Geometry: final body of the model. Coordinates: model frame, mm. Face numbers are marked on the shaded views. A direction names the side the tool comes from. Coordinates: 2 decimals unless noted, no trailing zeros. Loops run counter-clockwise (first coordinate to the right, second up) from the corner with the lowest first, then second, coordinate; pieces in that order, holes last. Notation, with made-up numbers: (79, -27) -> (103, -27) arc R17 cw to (103, -13) -> close; hole circle Ø2 at (59, 77.25). An arc over 180 degrees is marked (long way). One line per item, written item: value. Start each with the question number.
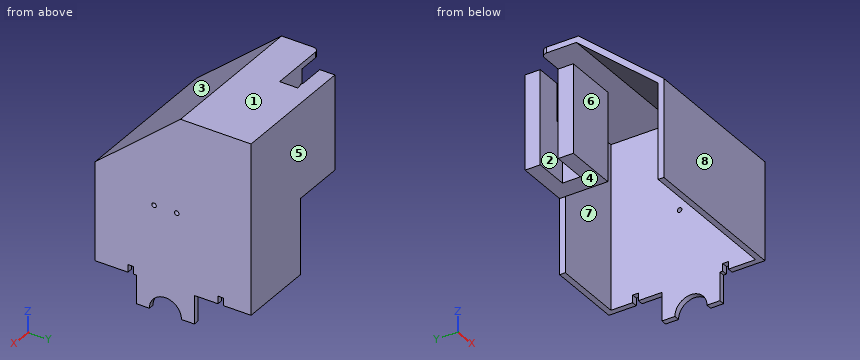
from build123d import *

# Parameters (mm, degrees)
BOSS_EXTRUDE1_DEPTH = 50
SKETCH2_W           = 3
SKETCH2_H           = 22.5
SKETCH2_W_2         = 40
SKETCH2_H_2         = 3
BOSS_EXTRUDE2_DEPTH = 40
SKETCH3_W           = 18
SKETCH3_H           = 9.5
CUT_EXTRUDE1_DEPTH  = 30
SKETCH4_W           = 3
SKETCH4_H           = 90
BOSS_EXTRUDE3_DEPTH = 79.5
SKETCH6_W           = 90
SKETCH6_H           = 3
BOSS_EXTRUDE4_DEPTH = 79
BOSS_EXTRUDE5_DEPTH = 3
FILLET1_R           = 3
SKETCH11_W          = 4
SKETCH11_H          = 3
CUT_EXTRUDE2_DEPTH  = 3
BOSS_EXTRUDE6_DEPTH = 3
SKETCH15_R          = 1.2
SKETCH15_W          = 4
SKETCH15_H          = 3
CUT_EXTRUDE3_DEPTH  = 3
CUT_EXTRUDE4_DEPTH  = 83
BOSS_EXTRUDE7_DEPTH = 82


with BuildPart() as part:
    # Sketch1 → Boss-Extrude1 (new body)
    with BuildSketch(Plane.XY.offset(75.054829109)):
        with BuildLine():
            Line((-97.212578399, 43.970791156), (-83.462578399, 43.970791156))
            ThreePointArc((-83.462578399, 43.970791156), (-82.462578399, 43.470791156), (-81.462578399, 43.970791156))
            Line((-81.462578399, 43.970791156), (-79.212578399, 43.970791156))
            Line((-79.212578399, 43.970791156), (-79.212578399, 34.470791156))
            Line((-79.212578399, 34.470791156), (-97.212578399, 34.470791156))
            Line((-97.212578399, 34.470791156), (-97.212578399, 26.470791156))
            Line((-97.212578399, 26.470791156), (-69.212578399, 26.470791156))
            Line((-69.212578399, 26.470791156), (-69.212578399, 51.970791156))
            Line((-69.212578399, 51.970791156), (-97.212578399, 51.970791156))
            Line((-97.212578399, 51.970791156), (-97.212578399, 43.970791156))
        make_face()
    extrude(amount=BOSS_EXTRUDE1_DEPTH)

    # Sketch2 → Boss-Extrude2 (add)
    with BuildSketch(Plane(origin=(-69.212578399, 0, 0), x_dir=(0, 0, -1), z_dir=(1, 0, 0))):
        with Locations((-123.554829109, 37.720791156)):
            Rectangle(SKETCH2_W, SKETCH2_H)
        Polygon((-75.054829109, 51.970791156), (-125.054829109, 51.970791156), (-125.054829109, 48.970791156), (-122.054829109, 48.970791156), (-75.054829109, 48.970791156), align=None)
        with Locations((-55.054829109, 50.470791156)):
            Rectangle(SKETCH2_W_2, SKETCH2_H_2)
    extrude(amount=BOSS_EXTRUDE2_DEPTH)

    # Sketch3 → Cut-Extrude1 (cut)
    with BuildSketch(Plane(origin=(0, 0, 75.054829109), x_dir=(-1, 0, 0), z_dir=(0, 0, -1))):
        with Locations((88.212578399, 39.220791156)):
            Rectangle(SKETCH3_W, SKETCH3_H)
    extrude(amount=-CUT_EXTRUDE1_DEPTH, mode=Mode.SUBTRACT)

    # Sketch4 → Boss-Extrude3 (add)
    with BuildSketch(Plane.XZ.offset(-48.970791156)):
        with Locations((-30.712578399, 80.054829109)):
            Rectangle(SKETCH4_W, SKETCH4_H)
    extrude(amount=BOSS_EXTRUDE3_DEPTH)

    # Sketch6 → Boss-Extrude4 (add)
    with BuildSketch(Plane.ZY.offset(32.212578399)):
        with Locations((80.054829109, -29.029208844)):
            Rectangle(SKETCH6_W, SKETCH6_H)
    extrude(amount=BOSS_EXTRUDE4_DEPTH)

    # Sketch7 → Boss-Extrude5 (add)
    with BuildSketch(Plane.XY.offset(125.054829109)):
        Polygon((-111.212578399, -27.529208844), (-32.212578399, -27.529208844), (-32.212578399, 26.470791156), (-97.212578399, 26.470791156), (-97.212578399, 34.470791156), (-111.212578399, 34.470791156), align=None)
    extrude(amount=-BOSS_EXTRUDE5_DEPTH)

    # Fillet1
    fillet1_edges = [part.edges().sort_by_distance(p)[0] for p in [
        (-111.212578399, 34.470791156, 123.554829109),
    ]]
    fillet(fillet1_edges, radius=FILLET1_R)

    # Sketch11 → Cut-Extrude2 (cut)
    with BuildSketch(Plane(origin=(-29.212578399, 0, 0), x_dir=(0, 0, -1), z_dir=(1, 0, 0))):
        with Locations((-37.054829109, 35.970791156)):
            Rectangle(SKETCH11_W, SKETCH11_H)
    extrude(amount=-CUT_EXTRUDE2_DEPTH, mode=Mode.SUBTRACT)

    # Sketch13 → Boss-Extrude6 (add)
    with BuildSketch(Plane(origin=(-29.212578399, 0, 0), x_dir=(0, 0, -1), z_dir=(1, 0, 0))):
        with BuildLine():
            Line((-20.054829109, 15.145791156), (-20.054829109, 21.970791156))
            Line((-20.054829109, 21.970791156), (-35.054829109, 21.970791156))
            Line((-35.054829109, 21.970791156), (-35.054829109, -8.679208844))
            Line((-35.054829109, -8.679208844), (-20.054829109, -8.679208844))
            Line((-20.054829109, -8.679208844), (-20.054829109, -1.854208844))
            ThreePointArc((-20.054829109, -1.854208844), (-28.554829109, 6.645791156), (-20.054829109, 15.145791156))
        make_face()
    extrude(amount=-BOSS_EXTRUDE6_DEPTH)

    # Sketch15 → Cut-Extrude3 (cut)
    with BuildSketch(Plane(origin=(-29.212578399, 0, 0), x_dir=(0, 0, -1), z_dir=(1, 0, 0))):
        with Locations((-75.054829109, 0.645791156)):
            Circle(SKETCH15_R)
        with Locations((-75.054829109, 12.645791156)):
            Circle(SKETCH15_R)
        with Locations((-37.054829109, -11.679208844)):
            Rectangle(SKETCH15_W, SKETCH15_H)
    extrude(amount=-CUT_EXTRUDE3_DEPTH, mode=Mode.SUBTRACT)

    # Sketch16 → Cut-Extrude4 (cut, through all)
    with BuildSketch(Plane(origin=(-29.212578399, 0, 0), x_dir=(0, 0, -1), z_dir=(1, 0, 0))):
        Polygon((-125.054829109, 16.970791156), (-85.054829109, -30.529208844), (-125.054829109, -30.529208844), align=None)
    extrude(amount=-CUT_EXTRUDE4_DEPTH, mode=Mode.SUBTRACT)

    # Sketch17 → Boss-Extrude7 (add)
    with BuildSketch(Plane(origin=(-29.212578399, 0, 0), x_dir=(0, 0, -1), z_dir=(1, 0, 0))):
        Polygon((-125.054829109, 19.299492846), (-125.054829109, 14.642089465), (-87.015841059, -30.529208844), (-83.093817159, -30.529208844), align=None)
    extrude(amount=-BOSS_EXTRUDE7_DEPTH)


solid = part.part
1. Section D-D on x = -49. Return the cut outline in (y, z).
2. Section C-C on z = 103. Return the cut outline in (x, y).
3. Set-up query: the marked faces 4, 5, 6, 7 and 8. Return all of +Z, -Z, +X, -X, +Y, -Y with unobstructed straight access to the full face (end or side cutting, diameter ignored); none if empty.
4. Draft query along Y for the marked faces 1, 2 and 3. Return one class per face: released by +Y, released by -Y, zero draft, split by the parting line, or undercut.
5. Section A-A on x = -100.5. Return the cut outline in (y, z), plus the area to 3 significant figures.
6. Section B-B on y = 29.5. Return the cut outline in (x, z), plus the area to 3 significant figures.
7. Line query: L1, parallel to Y at x = -93.5, z = 81; L2, parallel to Y at x = -54, z = 57.5; L3, parallel to X at y = 41.5, z = 102. Output: solid intervals per line, ascending. Write a range as [from, to].
8. Pin query (flat end, axial travel): pin 1 Ø2 at (y, z) = (25, 65) entering from -X; pin 2 Ø6.5 at (y, z) = (47.5, 106) entering from -X; pin 3 Ø14.5 at (x, z) = (-92, 100) entering from -Y; pin 4 Ø2 at (y, z) = (12.65, 75.05) entering from -X. Return the tip coordinate at first contact, or that it passes through.
Checks:
1. outline: (-30.53, 35.05) -> (-27.53, 35.05) -> (-27.53, 85.62) -> (15.74, 122.05) -> (48.97, 122.05) -> (48.97, 35.05) -> (51.97, 35.05) -> (51.97, 125.05) -> (14.64, 125.05) -> (-30.53, 87.02) -> close
2. outline: (-111.21, -11.55) -> (-29.21, -11.55) -> (-29.21, 51.97) -> (-97.21, 51.97) -> (-97.21, 43.97) -> (-79.21, 43.97) -> (-79.21, 34.47) -> (-97.21, 34.47) -> (-97.21, 26.47) -> (-69.21, 26.47) -> (-69.21, 48.97) -> (-32.21, 48.97) -> (-32.21, -6.89) -> (-111.21, -6.89) -> close
3. face 4: -Z, -X, +Y
3. face 5: +Z, -Z, +X, -X, +Y
3. face 6: -Z, -X
3. face 7: -Z
3. face 8: +Z, -Z, +X, -X, -Y
4. face 1: zero draft
4. face 2: undercut
4. face 3: released by -Y
5. outline: (-30.53, 35.05) -> (-27.53, 35.05) -> (-27.53, 85.62) -> (15.74, 122.05) -> (34.47, 122.05) -> (34.47, 125.05) -> (14.64, 125.05) -> (-30.53, 87.02) -> close
5. area: 385 mm²
6. outline: (-111.21, 122.05) -> (-97.21, 122.05) -> (-97.21, 75.05) -> (-69.21, 75.05) -> (-69.21, 122.05) -> (-32.21, 122.05) -> (-32.21, 35.05) -> (-29.21, 35.05) -> (-29.21, 125.05) -> (-111.21, 125.05) -> close
6. area: 1,820 mm²
7. L1: [-30.53, -27.53], [26.47, 34.47], [43.97, 51.97]
7. L2: [-30.53, -27.53], [48.97, 51.97]
7. L3: [-79.21, -69.21], [-32.21, -29.21]
8. pin 1: x = -32.21
8. pin 2: x = -97.21
8. pin 3: y = -23.72
8. pin 4: through
